Geometry: final body of the model. Coordinates: model frame, mm. Give positions to 0.01 mm unless a question says otherwise; leave off trailing zeros. Write each loop counter-clockwise with the first axis right and the second up, starting at its lowest first coordinate (ties: lowest second). Pieces come first, ordered by that corner, then holes.
Autodesk Inventor part; units mm, degrees
ref_plane "YZ Plane" through (0, 0, 0) normal (1, 0, 0) x (0, 1, 0)
ref_plane "XZ Plane" through (0, 0, 0) normal (0, 1, 0) x (-1, 0, 0)
ref_plane "XY Plane" through (0, 0, 0) normal (0, 0, 1) x (1, 0, 0)
sketch "Sketch1" plane through (0, 0, 0) normal (0, 0, 1) x (1, 0, 0)
  line L0 (-750, 51.5224) -> (750, 51.5224)
  line L1 (750, 51.5224) -> (750, 0)
  line L2 (750, 0) -> (-750, 0)
  line L3 (-750, 0) -> (-750, 51.5224)
  point P0 (0, 0)
  point P1 (0, 0)
  dimension "d0" = 1500
  dimension "d1" = 51.5224
extrude "Plate1" add sketch "Sketch1" along normal blind 3
sketch "Sketch2" plane through (750, 3, 0) normal (0, -1, 0) x (1, 0, 0)
  line L0 (-1500, 0) -> (0, 0)
  line L1 (0, 0) -> (0, 30)
  line L2 (0, 30) -> (-1500, 30)
  line L3 (-1500, 30) -> (-1500, 0)
edge flange "Flange1" height 30 angle 90 thickness 3 bend radius 3 thickness toward (0, -1, 0) relief tear relief width 3 relief depth 1.5 edges at (0, 0, 3) wall of the first edge with corners at (-750, 3, 0) (750, 3, 0) (750, 3, 30) (-750, 3, 30)
bend "Bend1"
corner "Corner1"
sketch "Sketch5" plane through (0, 0, 0) normal (0, 0, -1) x (-1, 0, 0)
  line L0 (750, 51.5224) -> (-750, 51.5224)
  line L1 (500, 51.5224) -> (500, 31)
  line L2 (500, 31) -> (503, 31)
  line L3 (503, 31) -> (503, 51.5224)
  line L4 (750, 0) -> (-750, 0)
  point P0 (0, 0)
  dimension "d18" = 3
  dimension "d19" = 247
  dimension "d20" = 31
extrude "Extrusion1" cut sketch "Sketch5" against normal through all
pattern_linear "Rectangular Pattern1" count 3 spacing 500 along (1, 0, 0) of "Extrusion1"
sketch "Sketch6" plane through (0, 0, 0) normal (0, 0, -1) x (-1, 0, 0)
  line L0 (-750, 51.5224) -> (-750, 6)
  circle A0 centre (-750, 51.5224) radius 15
  line L1 (-750, 51.5224) -> (-500, 51.5224)
  point P0 (0, 0)
  point P1 (-735, 51.5224)
  point P2 (-750, 36.5224)
  dimension "d24" = 30
extrude "Extrusion2" cut sketch "Sketch6" against normal through all contours L1 A0 L0 picked at (-740.1254, 50.4098)
mirror "Mirror1" about plane through (0, 0, 0) normal (1, 0, 0) of "Extrusion2"
equation "\"d1\" = Стрингер_5"
equation "\"d18\" = Thickness"
equation "\"d2\" = Thickness"
equation "\"d3\" = BendReliefWidth"
equation "\"d4\" = BendReliefDepth"
equation "\"d5\" = MinimumRemnant"
equation "\"d6\" = TransitionRadius"
equation "\"d9\" = BendRadius"
equation "\"d10\" = CornerReliefSize"
equation "\"d11\" = GapSize"
equation "\"d12\" = JacobiRadiusSize"
equation "\"BendRadius\" = Thickness"
equation "\"BendReliefWidth\" = Thickness"
equation "\"BendReliefDepth\" = 0.5 * Thickness"
equation "\"CornerReliefSize\" = 4 * Thickness"
equation "\"MinimumRemnant\" = 2 * Thickness"
equation "\"TransitionRadius\" = BendRadius"
equation "\"JacobiRadiusSize\" = BendRadius"
equation "\"GapSize\" = Thickness"
properties part number "МОО 055 стрингер борт 51"
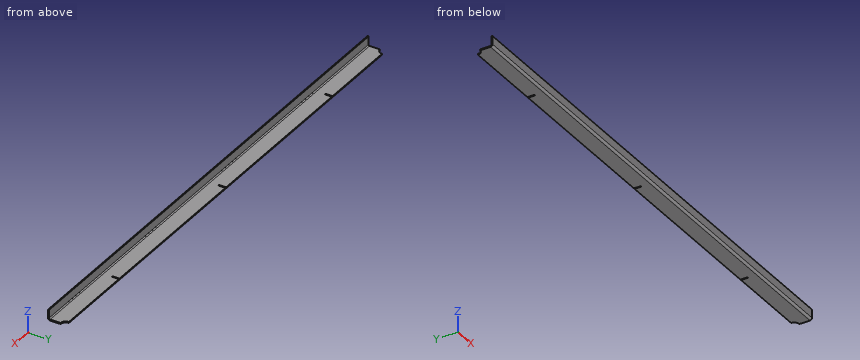
Q1. Ray query, line 1 along Z through (x, y) = (239, 28.5); line 2 along Y through (x, z) = (-119, 5). Return the intervals inside material, ascending.
Filled sheet:
line 1: z = 0 to 3
line 2: y = 0.08 to 3.17
Q2. Pin query (flat end, axial travel): P1, Ø2.5, axis at x = -501.5, z = 1, coming from the +Y side; P2, Ø2.5, axis at y = 40.5, z = 2, coming from the -X side; P3, Ø13.5, axis at x = 336, y = 34, coming from the +Z side. Return the tip coordinate at first contact, or that it passes through.
Filled sheet:
P1: stops at y = 31
P2: stops at x = -741.38
P3: stops at z = 3
Q3. Section A-A on x = -88.5. Output: boundary loops of the cut face in (y, z).
Filled sheet:
outline: (0, 6) arc R6 ccw to (6, 0) - (51.52, 0) - (51.52, 3) - (6, 3) arc R3 cw to (3, 6) - (3, 30) - (0, 30) - close
Q4. Section B-B on y = 18.5. Output: boundary loops of the cut face in (x, z).
Filled sheet:
outline: (-750, 0) - (750, 0) - (750, 3) - (-750, 3) - close
